```python
from build123d import *

# Parameters (mm, degrees)
BOSS_EXTRUDE1_DEPTH = 3
CUT_EXTRUDE4_DEPTH  = 10
CHAMFER1_SIZE       = 1
SKETCH4_R           = 2
CUT_EXTRUDE5_DEPTH  = 10


with BuildPart() as part:
    # Sketch3 → Boss-Extrude1 (new body)
    with BuildSketch(Plane.XY):
        Polygon((-26.921356186, 32.06604295), (27.378643814, 32.06604295), (31.378643814, 28.06604295), (31.378643814, -27.608755321), (27.378643814, -31.608755321), (-26.921356186, -31.608755321), (-30.921356186, -27.608755321), (-30.921356186, 28.06604295), align=None)
    extrude(amount=BOSS_EXTRUDE1_DEPTH)

    # Sketch2 → Cut-Extrude4 (cut)
    with BuildSketch(Plane.XY):
        Polygon((-11.874909576, 24.81604295), (-11.874909576, 23.81604295), (12.332197205, 23.81604295), (12.332197205, 24.81604295), (5.978643814, 31.16959634), (5.978643814, 32.31604295), (-5.521356186, 32.31604295), (-5.521356186, 31.16959634), align=None)
    extrude(amount=CUT_EXTRUDE4_DEPTH, mode=Mode.SUBTRACT)

    # Chamfer1
    chamfer1_edges = [part.edges().sort_by_distance(p)[0] for p in [
        (-16.221356186, 32.06604295, 3),
    ]]
    chamfer(chamfer1_edges, length=CHAMFER1_SIZE)
    chamfer1_2_edges = [part.edges().sort_by_distance(p)[0] for p in [
        (-29.421356186, 29.56604295, 3),
    ]]
    chamfer(chamfer1_2_edges, length=CHAMFER1_SIZE)
    chamfer1_3_edges = [part.edges().sort_by_distance(p)[0] for p in [
        (-30.921356186, -0.478462967, 3),
    ]]
    chamfer(chamfer1_3_edges, length=CHAMFER1_SIZE)
    chamfer1_4_edges = [part.edges().sort_by_distance(p)[0] for p in [
        (-28.421356186, -30.108755321, 3),
    ]]
    chamfer(chamfer1_4_edges, length=CHAMFER1_SIZE)
    chamfer1_5_edges = [part.edges().sort_by_distance(p)[0] for p in [
        (0.935750595, -31.608755321, 3),
    ]]
    chamfer(chamfer1_5_edges, length=CHAMFER1_SIZE)
    chamfer1_6_edges = [part.edges().sort_by_distance(p)[0] for p in [
        (29.878643814, -29.108755321, 3),
    ]]
    chamfer(chamfer1_6_edges, length=CHAMFER1_SIZE)
    chamfer1_7_edges = [part.edges().sort_by_distance(p)[0] for p in [
        (31.378643814, 0.935750595, 3),
    ]]
    chamfer(chamfer1_7_edges, length=CHAMFER1_SIZE)
    chamfer1_8_edges = [part.edges().sort_by_distance(p)[0] for p in [
        (28.878643814, 30.56604295, 3),
    ]]
    chamfer(chamfer1_8_edges, length=CHAMFER1_SIZE)
    chamfer1_9_edges = [part.edges().sort_by_distance(p)[0] for p in [
        (15.971537033, 32.06604295, 3),
    ]]
    chamfer(chamfer1_9_edges, length=CHAMFER1_SIZE)
    chamfer1_10_edges = [part.edges().sort_by_distance(p)[0] for p in [
        (9.207197205, 27.94104295, 3),
    ]]
    chamfer(chamfer1_10_edges, length=CHAMFER1_SIZE)
    chamfer1_11_edges = [part.edges().sort_by_distance(p)[0] for p in [
        (12.332197205, 24.31604295, 3),
    ]]
    chamfer(chamfer1_11_edges, length=CHAMFER1_SIZE)
    chamfer1_12_edges = [part.edges().sort_by_distance(p)[0] for p in [
        (0.228643814, 23.81604295, 3),
    ]]
    chamfer(chamfer1_12_edges, length=CHAMFER1_SIZE)
    chamfer1_13_edges = [part.edges().sort_by_distance(p)[0] for p in [
        (-11.874909576, 24.31604295, 3),
    ]]
    chamfer(chamfer1_13_edges, length=CHAMFER1_SIZE)
    chamfer1_14_edges = [part.edges().sort_by_distance(p)[0] for p in [
        (-8.749909576, 27.94104295, 3),
    ]]
    chamfer(chamfer1_14_edges, length=CHAMFER1_SIZE)

    # Sketch4 → Cut-Extrude5 (cut)
    with BuildSketch(Plane.XY.offset(3)):
        with Locations((-25, 27.31604295)):
            Circle(SKETCH4_R)
        with Locations(Location((25, 27.31604295, 0), (0, 0, 180))):
            Circle(SKETCH4_R)
        with Locations((25, -22.68395705)):
            Circle(SKETCH4_R)
        with Locations(Location((-25, -22.68395705, 0), (0, 0, 180))):
            Circle(SKETCH4_R)
    extrude(amount=-CUT_EXTRUDE5_DEPTH, mode=Mode.SUBTRACT)


solid = part.part
```
Design review of the part built by this model. Coordinates are the model's own, in mm. A direction names the side the tool comes from. Coordinates: 2 decimals unless noted, no trailing zeros. Loops run counter-clockwise (first coordinate to the right, second up) from the corner with the lowest first, then second, coordinate; pieces in that order, holes last. Notation, with made-up numbers: (16, 35) -> (34, 35) arc R16 cw to (34, 53) -> close; hole circle Ø7 at (55, 16). An arc over 180 degrees is marked (long way). Answer as a JSON object with one key per item and string values.
Q1. To check wall thickness, follow L1, parallel to Y at x = -25, z = 1.6; L2, parallel to X at y = 24, z = 0.5; L3, parallel to Y at x = -25, z = 2.4. State the ranges of each line that lie inside material, in increasing order.
Answer block:
{"L1": "y = -31.61 to -24.68, -20.68 to 25.32, 29.32 to 32.07", "L2": "x = -30.92 to -11.87, 12.33 to 31.38", "L3": "y = -31.21 to -24.68, -20.68 to 25.32, 29.32 to 31.67"}
Q2. Take a section at A-A on x = 25. Give the boundary of the cut face in (y, z), plus the area to 3 significant figures.
Answer block:
{"outline": "(-31.61, 0) -> (-24.68, 0) -> (-24.68, 3) -> (-30.61, 3) -> (-31.61, 2) -> close; (-20.68, 0) -> (25.32, 0) -> (25.32, 3) -> (-20.68, 3) -> close; (29.32, 0) -> (32.07, 0) -> (32.07, 2) -> (31.07, 3) -> (29.32, 3) -> close", "area": "166 mm^2"}
Q3. Tool access review of faces 1 (the flat face through (0, 23.816, 1)), 2 (the flat face through (9.568, 28.278, 2.493)), 3 (the flat face through (29.41, -29.58, 0.99)): name each direction out of +Z, -Z, +X, -X, +Y, -Y from which nothing blocks a thin tool from reaching the whole face with its end or side.
Answer block:
{"face 1": "+Z, -Z", "face 2": "+Z", "face 3": "+Z, -Z, +X, -Y"}
Q4. Take a section at B-B on x = -10.5. Give the boundary of the cut face in (y, z).
Answer block:
{"outline": "(-31.61, 0) -> (23.82, 0) -> (23.82, 2) -> (22.82, 3) -> (-30.61, 3) -> (-31.61, 2) -> close; (26.19, 0) -> (32.07, 0) -> (32.07, 2) -> (31.07, 3) -> (27.61, 3) -> (26.19, 2) -> close"}
Q5. Clearance check with flat-ended pins moving along their axes: pin 1 Ø12 at (x, y) = (-17, 25) entering from -Z; pin 2 Ø1.6 at (x, z) = (4.5, 1) entering from +Y. State where each tip first meets the part, or that it passes through.
Answer block:
{"pin 1": "stops at z = 0", "pin 2": "stops at y = 23.82"}
Q6. The part is to be moulded in two halves that separate along X. For faces 4 (the flat face through (29, 29.75, 2.49)), 5 (the flat face through (-28.95, 30.04, 0.99)), 6 (the cylindrical face through (27, 27.23, 1.52)), say which applies: +X half, -X half, draft (parallel to the pull), parting line (faces both ways), or undercut.
Answer block:
{"face 4": "+X half", "face 5": "-X half", "face 6": "undercut"}
Q7. Take a section at C-C on z = 1.4. Give the boundary of the cut face in (x, y).
Answer block:
{"outline": "(-30.92, -27.61) -> (-26.92, -31.61) -> (27.38, -31.61) -> (31.38, -27.61) -> (31.38, 28.07) -> (27.38, 32.07) -> (5.98, 32.07) -> (5.98, 31.17) -> (12.33, 24.82) -> (12.33, 23.82) -> (-11.87, 23.82) -> (-11.87, 24.82) -> (-5.52, 31.17) -> (-5.52, 32.07) -> (-26.92, 32.07) -> (-30.92, 28.07) -> close; hole circle Ø4 at (-25, -22.68); hole circle Ø4 at (-25, 27.32); hole circle Ø4 at (25, -22.68); hole circle Ø4 at (25, 27.32)"}
Q8. Take a section at D-D on x = 11. Give the boundary of the cut face in (y, z).
Answer block:
{"outline": "(-31.61, 0) -> (23.82, 0) -> (23.82, 2) -> (22.82, 3) -> (-30.61, 3) -> (-31.61, 2) -> close; (26.15, 0) -> (32.07, 0) -> (32.07, 2) -> (31.07, 3) -> (27.56, 3) -> (26.15, 2) -> close"}
